from build123d import *

# Parameters (mm, degrees)
SKETCH1_W         = 28
SKETCH1_H         = 1
DOME1_FACE_RADIUS = 1
DOME1_HEIGHT      = 1
DOME2_FACE_RADIUS = 1
DOME2_HEIGHT      = 1


with BuildPart() as part:
    # Sketch1 → Revolve1 (revolve)
    with BuildSketch(Plane.XY):
        with Locations((0, 0.5)):
            Rectangle(SKETCH1_W, SKETCH1_H)
    revolve(axis=Axis((-14, 0, 0), (1, 0, 0)))

    # Dome1: a dome of height H over a round flat face of radius A is a cap of a sphere of radius (A * A + H * H) / (2 * H)
    dome1_r = (DOME1_FACE_RADIUS * DOME1_FACE_RADIUS + DOME1_HEIGHT * DOME1_HEIGHT) / (2 * DOME1_HEIGHT)
    dome1_base = Plane((-14, 0, 0), z_dir=(-1, 0, 0))
    with Locations(dome1_base.offset(DOME1_HEIGHT - dome1_r)):
        dome1_ball = Sphere(dome1_r, mode=Mode.PRIVATE)
    add(split(dome1_ball, bisect_by=dome1_base, keep=Keep.TOP, mode=Mode.PRIVATE))

    # Dome2: a dome of height H over a round flat face of radius A is a cap of a sphere of radius (A * A + H * H) / (2 * H)
    dome2_r = (DOME2_FACE_RADIUS * DOME2_FACE_RADIUS + DOME2_HEIGHT * DOME2_HEIGHT) / (2 * DOME2_HEIGHT)
    dome2_base = Plane((14, 0, 0), z_dir=(1, 0, 0))
    with Locations(dome2_base.offset(DOME2_HEIGHT - dome2_r)):
        dome2_ball = Sphere(dome2_r, mode=Mode.PRIVATE)
    add(split(dome2_ball, bisect_by=dome2_base, keep=Keep.TOP, mode=Mode.PRIVATE))


solid = part.part
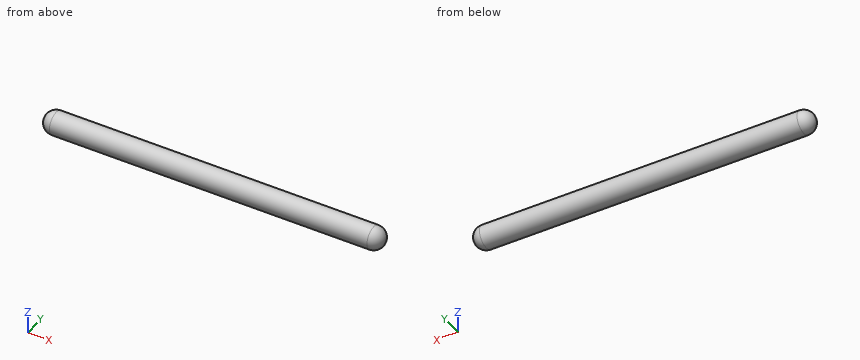
For this review, take the finished solid that the model builds, in its own axes (mm). Round coordinates to 2 decimals unless told otherwise and drop trailing zeros. Order: outer loops, then holes, each group sorted by start corner. A loop starts at its lowest first (then second) coordinate and runs counter-clockwise, first axis right, second up. Notation, with made-up numbers: M 74.5,-14 L 102.5,-14 A25 cw 102.5,3 Z; hole C -27.5,0.5 d5. An arc over 180 degrees is marked long. Use a Markdown table: item, result. Add a question column.
Item 1: Add section B-B, the plane y = 0.25. Give the boundary of the cut face in (x, z).
Item 2: Add section A-A, the plane z = -0.6. Give the boundary of the cut face in (x, y).
Item 3: Insertion check: pin 1 (1 mm diameter, centred on x = 4.5, z = -1, fed in from -Y). The pin has a flat end and moves straight along its axis. Give the tip position at first contact, or say it passes through.
Item 4: To check wall thickness, follow line 1 along Y through (x, z) = (11.5, -0.05); line 2 along Z through (x, y) = (6.5, -0.1); line 3 along X through (y, z) = (-0.35, -0.2). State the ranges of each line that lie inside material, in increasing order.
Geometry results:
| question | item | result |
|---|---|---|
| 1 | outline | M -14,-0.97 L 14,-0.97 A0.97 ccw 14,0.97 L -14,0.97 A0.97 ccw Z |
| 2 | outline | M -14,-0.8 L 14,-0.8 A0.8 ccw 14,0.8 L -14,0.8 A0.8 ccw Z |
| 3 | pin 1 | stops at y = -0.87 |
| 4 | line 1 | y = -1 to 1 |
| 4 | line 2 | z = -0.99 to 0.99 |
| 4 | line 3 | x = -14.92 to 14.92 |
